```python
from build123d import *

# Parameters (mm, degrees)
CROQUIS1_W            = 112
CROQUIS1_H            = 140
BRIDA_BASE1_DEPTH     = 0.5
CORTAR_EXTRUIR1_DEPTH = 10
CROQUIS6_R            = 1.5
CORTAR_EXTRUIR2_DEPTH = 10
CROQUIS7_R            = 1.5
CORTAR_EXTRUIR3_DEPTH = 10


# Sheet-metal steps are written as plain solids
with BuildPart() as part:
    # Croquis1 → Brida base1 (new body)
    with BuildSketch(Plane(origin=(0, 0, 0), x_dir=(1, 0, 0), z_dir=(0, 1, 0))):
        Rectangle(CROQUIS1_W, CROQUIS1_H)
    extrude(amount=-BRIDA_BASE1_DEPTH)

    # Croquis5 → Cortar-Extruir1 (cut)
    with BuildSketch(Plane(origin=(0, 0, 0), x_dir=(1, 0, 0), z_dir=(0, 1, 0))):
        Polygon((-15.25, 57), (-15.25, 70), (-56, 70), (-56, 50), (-50.5, 50), (-50.5, 58), (-31, 58), (-31, 50), (-25.5, 50), (-25.5, 57), align=None)
        Polygon((56, 70), (15.25, 70), (15.25, 57), (25.5, 57), (25.5, 50), (31, 50), (31, 58), (50.5, 58), (50.5, 50), (56, 50), align=None)
    extrude(amount=-CORTAR_EXTRUIR1_DEPTH, mode=Mode.SUBTRACT)

    # Croquis6 → Cortar-Extruir2 (cut)
    with BuildSketch(Plane(origin=(0, 0, 0), x_dir=(1, 0, 0), z_dir=(0, 1, 0))):
        with Locations(Location((-40.75, 54.125, 0), (0, 0, 270))):
            Circle(CROQUIS6_R)
        with Locations(Location((0, 66.125, 0), (0, 0, 270))):
            Circle(CROQUIS6_R)
        with Locations(Location((40.75, 54.125, 0), (0, 0, 90))):
            Circle(CROQUIS6_R)
    extrude(amount=-CORTAR_EXTRUIR2_DEPTH, mode=Mode.SUBTRACT)

    # Croquis7 → Cortar-Extruir3 (cut)
    with BuildSketch(Plane(origin=(0, 0, 0), x_dir=(1, 0, 0), z_dir=(0, 1, 0))):
        with Locations(Location((-16, -38.5, 0), (0, 0, 270))):
            Circle(CROQUIS7_R)
        with Locations(Location((-16, -46.5, 0), (0, 0, 90))):
            Circle(CROQUIS7_R)
        with Locations(Location((-10, -64.5, 0), (0, 0, 270))):
            Circle(CROQUIS7_R)
        with Locations(Location((-30, -64.5, 0), (0, 0, 270))):
            Circle(CROQUIS7_R)
        with Locations(Location((30, -64.5, 0), (0, 0, 90))):
            Circle(CROQUIS7_R)
        with Locations(Location((10, -64.5, 0), (0, 0, 90))):
            Circle(CROQUIS7_R)
        with Locations(Location((-51, -64.5, 0), (0, 0, 270))):
            Circle(CROQUIS7_R)
        with Locations(Location((51, -64.5, 0), (0, 0, 90))):
            Circle(CROQUIS7_R)
    extrude(amount=-CORTAR_EXTRUIR3_DEPTH, mode=Mode.SUBTRACT)


solid = part.part
```
Model file for the job. Use its own axes, mm. Round coordinates to 2 decimals unless told otherwise and drop trailing zeros. Write each loop counter-clockwise with the first axis right and the second up, starting at its lowest first coordinate (ties: lowest second). Pieces come first, ordered by that corner, then holes. Notation, with made-up numbers: M 25.5,-29.75 L 65.5,-29.75 A19 ccw 65.5,-10.75 Z; hole C -32.5,-14.75 d10. An arc over 180 degrees is marked long. Put each result on its own line as item: value.
Item 1: Cut at B-B (z = 46.5). List the corners of the cut face in (x, y), and give its area (3 significant figures).
Responses:
outline: M -56,-0.5 L -17.5,-0.5 L -17.5,0 L -56,0 Z; M -14.5,-0.5 L 56,-0.5 L 56,0 L -14.5,0 Z
area: 54.5 mm²
Item 2: Cut at C-C (y = -0.25). State how many separate pieces and enclosed holes the cut face has, and give its area (3 significant figures).
Responses:
separate pieces: 1
enclosed holes: 11
area: 14,400 mm²
Item 3: Cut at D-D (x = -19). List the corners of the cut face in (y, z), and give its area (3 significant figures).
Responses:
outline: M -0.5,-57 L 0,-57 L 0,70 L -0.5,70 Z
area: 63.5 mm²
Item 4: Probe L1, parallel to X at y = -0.4, z = -52; L2, parallel to Z at x = 51, y = -0.1; L3, parallel to Z at x = -33, y = -0.1. List the from-to ranges inside material, lowest first. Write a range as from..to.
Responses:
L1: -50.5..-31, -25.5..25.5, 31..50.5
L2: -50..63, 66..70
L3: -58..70
Item 5: Mould opens along X. For faces 1 (the flat face through (-1, 0, -1)), 2 (the cylindrical face through (-29.55, -0.25, 65.93)) say: +X half, -X half, draft (parallel to the pull), parting line (faces both ways), or undercut.
Responses:
face 1: draft
face 2: undercut
Item 6: Cut at A-A (x = 10). List the corners of the cut face in (y, z), and give its area (3 significant figures).
Responses:
outline: M -0.5,-70 L 0,-70 L 0,63 L -0.5,63 Z; M -0.5,66 L 0,66 L 0,70 L -0.5,70 Z
area: 68.5 mm²
